```python
from build123d import *

# Parameters (mm, degrees)
SKETCH1_W           = 594
SKETCH1_H           = 400
SKETCH1_R           = 12.25
BOSS_EXTRUDE1_DEPTH = 18
SKETCH2_R           = 16.5
CUT_EXTRUDE1_DEPTH  = 9.525
SKETCH3_R           = 4
CUT_EXTRUDE2_DEPTH  = 80
SKETCH4_R           = 2.38125
CUT_EXTRUDE3_DEPTH  = 9.525


with BuildPart() as part:
    # Sketch1 → Boss-Extrude1 (new body)
    with BuildSketch(Plane.XY):
        Rectangle(SKETCH1_W, SKETCH1_H)
        with Locations((252, 28.55)):
            Circle(SKETCH1_R, mode=Mode.SUBTRACT)
        with Locations((-252, 125)):
            Circle(SKETCH1_R, mode=Mode.SUBTRACT)
        with Locations((-252, 80)):
            Circle(SKETCH1_R, mode=Mode.SUBTRACT)
        with Locations((-252, 35)):
            Circle(SKETCH1_R, mode=Mode.SUBTRACT)
        with Locations((-252, -10)):
            Circle(SKETCH1_R, mode=Mode.SUBTRACT)
        with BuildLine():
            Line((-137, -105.42), (132, -105.42))
            ThreePointArc((132, -105.42), (144.727922061, -100.147922061), (150, -87.42))
            Line((150, -87.42), (150, 137.08))
            ThreePointArc((150, 137.08), (144.727922061, 149.807922061), (132, 155.08))
            Line((132, 155.08), (-137, 155.08))
            ThreePointArc((-137, 155.08), (-149.727922061, 149.807922061), (-155, 137.08))
            Line((-155, 137.08), (-155, -87.42))
            ThreePointArc((-155, -87.42), (-149.727922061, -100.147922061), (-137, -105.42))
        make_face(mode=Mode.SUBTRACT)
        with BuildLine():
            Line((254.386023622, 145.979320454), (270.808070866, 141.845754885))
            ThreePointArc((270.808070866, 141.845754885), (274.565595901, 138.584722637), (274.166216108, 133.625506823))
            Line((274.166216108, 133.625506823), (256.703716108, 105.050506823))
            ThreePointArc((256.703716108, 105.050506823), (252, 102.4125), (247.296283892, 105.050506823))
            Line((247.296283892, 105.050506823), (229.833783892, 133.625506823))
            ThreePointArc((229.833783892, 133.625506823), (229.434404099, 138.584722637), (233.191929134, 141.845754885))
            Line((233.191929134, 141.845754885), (249.613976378, 145.979320454))
            ThreePointArc((249.613976378, 145.979320454), (252, 146.275), (254.386023622, 145.979320454))
        make_face(mode=Mode.SUBTRACT)
    extrude(amount=BOSS_EXTRUDE1_DEPTH)

    # Sketch2 → Cut-Extrude1 (cut)
    with BuildSketch(Plane.XY.offset(18)):
        with Locations((-252, 125)):
            Circle(SKETCH2_R)
        with Locations((-252, 80)):
            Circle(SKETCH2_R)
        with Locations((-252, 35)):
            Circle(SKETCH2_R)
        with Locations((-252, -10)):
            Circle(SKETCH2_R)
    extrude(amount=-CUT_EXTRUDE1_DEPTH, mode=Mode.SUBTRACT)

    # Sketch3 → Cut-Extrude2 (cut)
    with BuildSketch(Plane.XY.offset(18)):
        with Locations((0, 165.075)):
            Circle(SKETCH3_R)
        with Locations((-233.3625, 165.075)):
            Circle(SKETCH3_R)
        with Locations((179.3875, 165.075)):
            Circle(SKETCH3_R)
        with Locations((0, -115.42)):
            Circle(SKETCH3_R)
        with Locations((-165, 24.83)):
            Circle(SKETCH3_R)
        with Locations((160, 24.83)):
            Circle(SKETCH3_R)
    extrude(amount=-CUT_EXTRUDE2_DEPTH, mode=Mode.SUBTRACT)

    # Sketch4 → Cut-Extrude3 (cut)
    with BuildSketch(Plane.XY.offset(18)):
        with Locations((252, 47.6)):
            Circle(SKETCH4_R)
        with Locations((252, 9.5)):
            Circle(SKETCH4_R)
    extrude(amount=-CUT_EXTRUDE3_DEPTH, mode=Mode.SUBTRACT)


solid = part.part
```
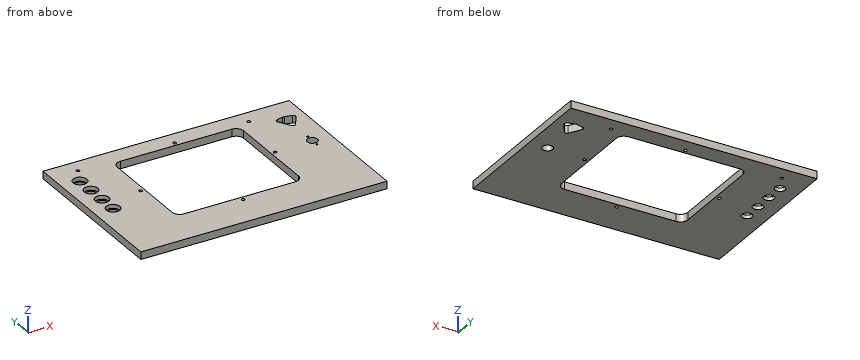
Here's how the part is built. I have some questions about the finished solid (model axes, mm). Coordinates: 2 decimals unless noted, no trailing zeros. Write each loop counter-clockwise with the first axis right and the second up, starting at its lowest first coordinate (ties: lowest second). Pieces come first, ordered by that corner, then holes. Notation, with made-up numbers: (50, -13) -> (107, -13) arc R25 ccw to (107, 26) -> close; hole circle Ø4 at (-38, 42). An arc over 180 degrees is marked (long way). Use a Markdown table: item, result. Add a question column.
(1) If we section it at B-B, the plane y = 80: Write out the boundary of the cut face in (x, z) (3 decimals), and give its area (3 significant figures).
(2) Please list where these lines run through material, in increasing order: line 1 (Y direction, x = -1, z = 5.25); line 2 (Y direction, x = 252, z = 11.75) (1 decimal); line 3 (Y direction, x = 0, z = 11.5) (3 decimals).
(3) I'm going to push a flat-ended pin straight in: P1, Ø22, axis at x = -252, y = 80, coming from the -Z side. Where does the tip first touch, or does it pass through?
(4) If we section it at C-C, the plane z = 13: State how many separate pieces and enclosed holes the cut face has, and give its area (3 significant figures).
(5) If we section it at A-A, the plane x = 81: Write out the boundary of the cut face in (y, z), and give its area (3 significant figures).
Outcome:
| question | item | result |
|---|---|---|
| 1 | outline | (-297, 0) -> (-264.25, 0) -> (-264.25, 8.475) -> (-268.5, 8.475) -> (-268.5, 18) -> (-297, 18) -> close; (-239.75, 0) -> (-155, 0) -> (-155, 18) -> (-235.5, 18) -> (-235.5, 8.475) -> (-239.75, 8.475) -> close; (150, 0) -> (297, 0) -> (297, 18) -> (150, 18) -> close |
| 1 | area | 4,680 mm^2 |
| 2 | line 1 | y = -200 to -119.29, -111.55 to -105.42, 155.08 to 161.2, 168.95 to 200 |
| 2 | line 2 | y = -200 to 7.1, 11.9 to 16.3, 40.8 to 45.2, 50 to 102.4, 146.3 to 200 |
| 2 | line 3 | y = -200 to -119.42, -111.42 to -105.42, 155.08 to 161.075, 169.075 to 200 |
| 3 | P1 | passes through |
| 4 | separate pieces | 1 |
| 4 | enclosed holes | 15 |
| 4 | area | 153,000 mm^2 |
| 5 | outline | (-200, 0) -> (-105.42, 0) -> (-105.42, 18) -> (-200, 18) -> close; (155.08, 0) -> (200, 0) -> (200, 18) -> (155.08, 18) -> close |
| 5 | area | 2,510 mm^2 |
